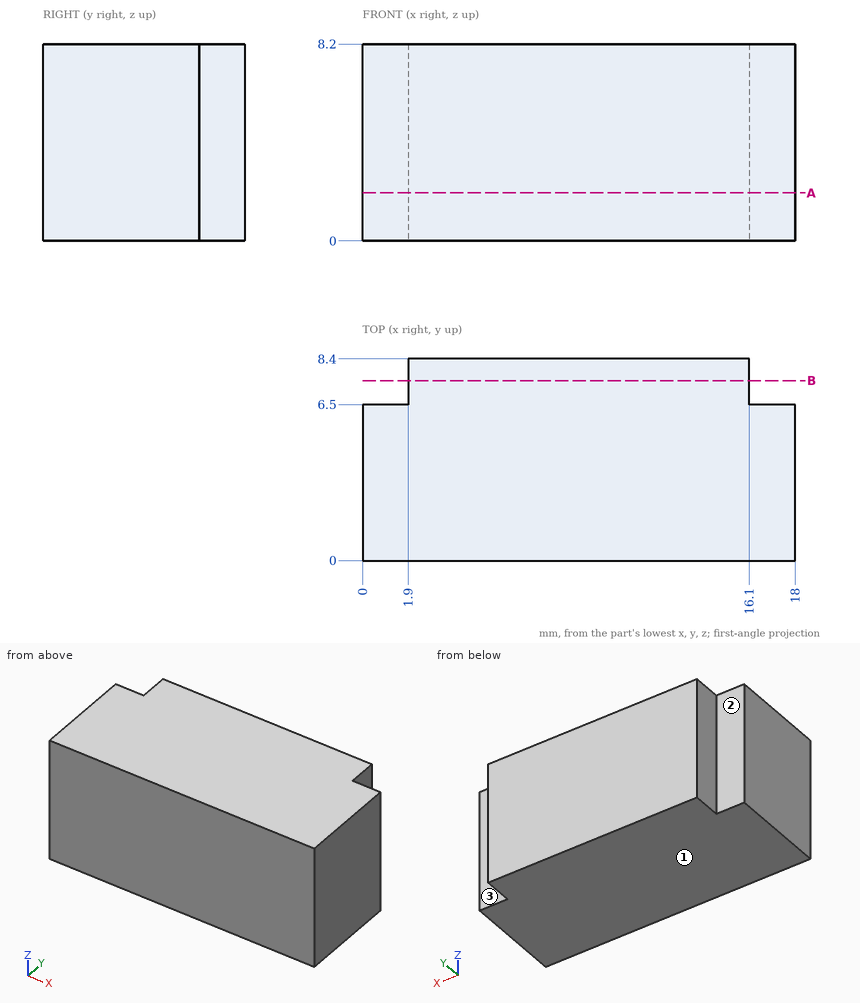
Design review of the part shown in the three views and the two pictorial views. Dimensions are in mm from the part's minimum x, y and z. A direction names the side the tool comes from. Give positions to 0.01 mm unless a question says otherwise; leave off trailing zeros. Loops run counter-clockwise (first coordinate to the right, second up) from the corner with the lowest first, then second, coordinate; pieces in that order, holes last. Notation, with made-up numbers: (-35, -13.5) -> (5, -13.5) arc R19 ccw to (5, 15.5) -> close; hole circle Ø7 at (-38, 64). An arc over 180 degrees is marked (long way). One line per question, with ' | ' between items.
1) We need section B-B (y = 7.5). Write out the cut boundary in (x, z), plus the area to 3 significant figures.
Resolved:
outline: (1.9, 0) -> (16.1, 0) -> (16.1, 8.2) -> (1.9, 8.2) -> close | area: 116 mm2
2) To check wall thickness, follow probe 1 along Y at (x, z) = (17.25, 6.25); probe 2 along X at (y, z) = (7, 2.5). State the ranges of each line that lie inside material, in increasing order.
Resolved:
probe 1: y = 0 to 6.5 | probe 2: x = 1.9 to 16.1
3) Insertion check: pin 1 Ø1.5 at (y, z) = (8, 5.5) entering from -X; pin 2 Ø0.6 at (x, z) = (17, 3) entering from +Y; pin 3 Ø0.6 at (y, z) = (7.5, 2.5) entering from +X. Each pin has a flat end and moves straight along its axis. Give the tip position at first contact, or say it passes through.
Resolved:
pin 1: stops at x = 1.9 | pin 2: stops at y = 6.5 | pin 3: stops at x = 16.1
4) For the marked faces 1, 2 and 3, list the 3-axis set-ups (+Z, -Z, +X, -X, +Y, -Y) from which the entire face can be reached by the end or side of a thin tool; tool diameter is ignored.
Resolved:
face 1: -Z, +X, -X, +Y, -Y | face 2: +Z, -Z, -X, +Y | face 3: +Z, -Z, +X, +Y
5) We need section A-A (z = 2). Write out the cut boundary in (x, y), plus the area to 3 significant figures.
Resolved:
outline: (0, 0) -> (18, 0) -> (18, 6.5) -> (16.1, 6.5) -> (16.1, 8.4) -> (1.9, 8.4) -> (1.9, 6.5) -> (0, 6.5) -> close | area: 144 mm2
